The model under review builds one solid part; all positions refer to its coordinate system, in mm. Face numbers are marked on the shaded views. Round coordinates to 2 decimals unless told otherwise and drop trailing zeros. Order: outer loops, then holes, each group sorted by start corner. A loop starts at its lowest first (then second) coordinate and runs counter-clockwise, first axis right, second up. Notation, with made-up numbers: (3.5, 7) - (22.5, 7) arc R21 cw to (22.5, 29) - close; hole circle Ø8 at (48, 16). An arc over 180 degrees is marked (long way). One line per question, with ' | ' between items. Start each with the question number.
Item 1: Add section C-C on x = 243. State the section outline as (y, z) points, and give its area (3 significant figures).
Item 2: Draft analysis for pull direction X (two halves, no side actions). For the marked faces 1, 2 and 3, state which applies: +X half, -X half, draft (parallel to the pull), parting line (faces both ways), or undercut.
Item 3: Add section B-B on x = 55. State the section outline as (y, z) points.
Item 4: Insertion check: pin 1 Ø10 at (x, y) = (158.5, -2) entering from -Z; pin 2 Ø2 at (x, y) = (225.5, -7) entering from +Z; pin 3 Ø6 at (x, z) = (210, -12) entering from +Y; pin 4 Ø8 at (x, z) = (49.5, 13.5) entering from +Y. Each pin has a flat end and moves straight along its axis. Give the tip position at first contact, or say it passes through.
Item 5: For L1, parallel to Z at x = 201.5, y = -10; L2, parallel to Y at x = 186.5, z = -0.5; L3, parallel to X at y = -9, z = -3.5, list the stretches that pass through material, from the lowest coordinate up. Write a range as [from, to].
Item 6: Add section A-A on x = 203. State the section outline as (y, z) points, and give its area (3 significant figures).
from build123d import *

# Parameters (mm, degrees)
CUT_EXTRUDE2_DEPTH = 25.4


with BuildPart() as part:
    # Sketch1 → Revolve6 (revolve)
    with BuildSketch(Plane.XY, mode=Mode.PRIVATE) as revolve6_sk:
        with BuildLine():
            Line((6.927857085, 8.89), (57.727857085, 8.89))
            ThreePointArc((57.727857085, 8.89), (68.726379713, 2.54), (79.724902341, 8.89))
            Line((79.724902341, 8.89), (84.804902341, 8.89))
            Line((84.804902341, 8.89), (84.804902341, -3.81))
            Line((84.804902341, -3.81), (211.804902341, -3.81))
            Line((211.804902341, -3.81), (237.204902341, 2.54))
            Line((237.204902341, 2.54), (262.604902341, -3.81))
            Line((262.604902341, -3.81), (262.604902341, -10.16))
            Line((262.604902341, -10.16), (-5.206352051, -10.16))
            ThreePointArc((-5.206352051, -10.16), (-4.365299375, 2.693819245), (6.927857085, 8.89))
        make_face()
    revolve(revolve6_sk.sketch.rotate(Axis((-5.206352051, -10.16, 0), (1, 0, 0)), 180), axis=Axis((-5.206352051, -10.16, 0), (1, 0, 0)))

    # Sketch3 → Cut-Extrude2 (cut, symmetric)
    with BuildSketch(Plane.XY):
        Polygon((211.804902341, -3.81), (262.604902341, -7.62), (262.604902341, 19.982961782), (211.804902341, 19.982961782), align=None)
        Polygon((262.604902341, -40.302961782), (262.604902341, -12.7), (211.804902341, -16.51), (211.804902341, -40.302961782), align=None)
    extrude(amount=CUT_EXTRUDE2_DEPTH, both=True, mode=Mode.SUBTRACT)


solid = part.part
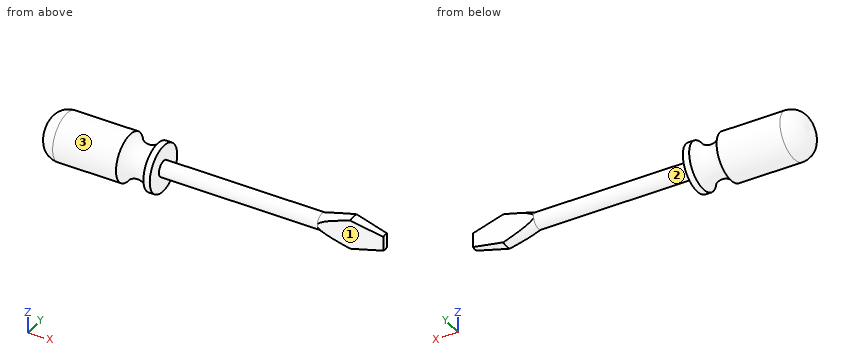
Determined:
1) outline: (-14.17, -10.51) arc R11.25 ccw to (-6.15, -10.51) - (-6.15, 10.51) arc R11.25 ccw to (-14.17, 10.51) - close | area: 177 mm2
2) face 1: +X half | face 2: undercut | face 3: draft
3) outline: circle Ø38.1 at (-10.16, 0)
4) pin 1: z = -5.51 | pin 2: z = 9.64 | pin 3: through | pin 4: y = 6.35
5) L1: [-6.35, 6.35] | L2: [-16.49, -3.83] | L3: [-6.32, 262.6]
6) outline: circle Ø12.7 at (-10.16, 0) | area: 127 mm2
